Here's how the part is built. I have some questions about the finished solid (model axes, mm). A direction names the side the tool comes from. Round coordinates to 2 decimals unless told otherwise and drop trailing zeros. Order: outer loops, then holes, each group sorted by start corner. A loop starts at its lowest first (then second) coordinate and runs counter-clockwise, first axis right, second up. Notation, with made-up numbers: (-26.5, -7.75) - (18.5, -7.75) arc R10 cw to (18.5, 2.25) - close; hole circle Ø5 at (68.25, -18). An arc over 180 degrees is marked (long way). Answer as a JSON object with one key per item and string values.
```python
from build123d import *

# Parameters (mm, degrees)
SKETCH_W           = 42.3
SKETCH_H           = 42.3
PAD_DEPTH          = 38
SKETCH001_R        = 11.4
PAD001_DEPTH       = 40
SKETCH002_R        = 2.5
PAD002_DEPTH       = 61.5
CHAMFER_SIZE       = 5
SKETCH003_W        = 10
SKETCH003_H        = 3
POCKET_DEPTH       = 18
SKETCH004_W        = 16.2
SKETCH004_H        = 27.15
PAD003_DEPTH       = 9.4
SKETCH005_R        = 2.25
POCKET001_DEPTH    = 4.5
POLARPATTERN_COUNT = 4


with BuildPart() as part:
    # Sketch → Pad (new body)
    with BuildSketch(Plane.XY):
        Rectangle(SKETCH_W, SKETCH_H)
    extrude(amount=PAD_DEPTH)

    # Sketch001 → Pad001 (join)
    with BuildSketch(Plane.XY):
        Circle(SKETCH001_R)
    extrude(amount=PAD001_DEPTH)

    # Sketch002 → Pad002 (join)
    with BuildSketch(Plane.XY):
        Circle(SKETCH002_R)
    extrude(amount=PAD002_DEPTH)

    # Chamfer
    chamfer_edges = [part.edges().sort_by_distance(p)[0] for p in [
        (-21.15, 21.15, 19),
        (-21.15, -21.15, 19),
        (21.15, 21.15, 19),
        (21.15, -21.15, 19),
    ]]
    chamfer(chamfer_edges, length=CHAMFER_SIZE)

    # Sketch003 (on Face16 of Chamfer) → Pocket (cut)
    with BuildSketch(Plane.XY.offset(61.5)):
        with Locations((0, 3.5)):
            Rectangle(SKETCH003_W, SKETCH003_H)
    extrude(amount=-POCKET_DEPTH, mode=Mode.SUBTRACT)

    # Sketch004 → Pad003 (join)
    with BuildSketch(Plane.XY):
        with Locations((0, 13.575)):
            Rectangle(SKETCH004_W, SKETCH004_H)
    extrude(amount=PAD003_DEPTH)

    # Sketch005 (on Face5 of Pad003) → Pocket001 (cut)
    with BuildSketch(Plane.XY.offset(38)):
        with Locations((-15.5, 16.484926)):
            Circle(SKETCH005_R)
    pocket001 = extrude(amount=-POCKET001_DEPTH, mode=Mode.SUBTRACT)

    # PolarPattern: Pocket001 ×4 about axis
    polarpattern_axis = Axis((0, 0, 38), (0, 0, 1))
    for i in range(1, POLARPATTERN_COUNT):
        add(pocket001.rotate(polarpattern_axis, i * 360 / POLARPATTERN_COUNT), mode=Mode.SUBTRACT)


solid = part.part
```
1. Imagine slicing it at A-A (z = 6). List the corners of the cut face in (x, y) for me, plus the area to 3 significant figures.
Responses:
{"outline": "(-21.15, -16.15) - (-16.15, -21.15) - (16.15, -21.15) - (21.15, -16.15) - (21.15, 16.15) - (16.15, 21.15) - (8.1, 21.15) - (8.1, 27.15) - (-8.1, 27.15) - (-8.1, 21.15) - (-16.15, 21.15) - (-21.15, 16.15) - close", "area": "1,840 mm2"}
2. Imagine slicing it at B-B (y = -10). List the corners of the cut face in (x, z) for me, plus the area to 3 significant figures.
Responses:
{"outline": "(-21.15, 0) - (21.15, 0) - (21.15, 38) - (5.47, 38) - (5.47, 40) - (-5.47, 40) - (-5.47, 38) - (-21.15, 38) - close", "area": "1,630 mm2"}
3. For faces 1 (the face through (0, 2, 53)), 2 (the face through (0, 3, 0)), 3 (the face through (18.38, 14.29, 35.78)), 4 (the face through (8.1, 24, 5)), 5 (the face through (-8.1, 24, 5)), which set-ups out of +Z, -Z, +X, -X, +Y, -Y let a thin tool reach every point of the face, with its end or its side?
Responses:
{"face 1": "+Z, +X, -X, +Y", "face 2": "-Z, +X, -X, +Y, -Y", "face 3": "+Z", "face 4": "+Z, -Z, +X, +Y", "face 5": "+Z, -Z, -X, +Y"}
4. Thinking about a two-plate mould opening in X: for faces 6 (the face through (-17, -16, 33.5)), 7 (the face through (14.29, -18.38, 35.78)), 8 (the face through (9, -9, 38)), 9 (the face through (18.7, 18.6, 18.7)), which applies, pulls with the +X half, pulls with the -X half, needs draft (parallel to the pull), parting line crosses it, or undercut?
Responses:
{"face 6": "undercut", "face 7": "undercut", "face 8": "needs draft", "face 9": "pulls with the +X half"}
5. For P1, Ø1.8, axis at x = -1.5, y = 23, coming from the +Z side; P2, Ø3.5, axis at x = 0.5, z = 53, coming from the +Y side; P3, Ø1.5, axis at x = -3.5, y = 9, coming from the +Z side; P4, Ø5, axis at y = 5.5, z = 54.5, coming from the +X side, each with a flat end and sliding along its axis, tell me the tip position at first contact or that it passes through.
Responses:
{"P1": "z = 9.4", "P2": "y = 2", "P3": "z = 40", "P4": "through"}
6. Imagine slicing it at C-C (x = 0). List the corners of the cut face in (y, z) for me.
Responses:
{"outline": "(-21.15, 0) - (27.15, 0) - (27.15, 9.4) - (21.15, 9.4) - (21.15, 38) - (11.4, 38) - (11.4, 40) - (2.5, 40) - (2.5, 43.5) - (2, 43.5) - (2, 61.5) - (-2.5, 61.5) - (-2.5, 40) - (-11.4, 40) - (-11.4, 38) - (-21.15, 38) - close"}
7. If I drill on L1, parallel to Y at x = -17.5, z = 34; L2, parallel to X at y = -15, z = 36; L3, parallel to Z at x = 16, y = -4, over which ranges is the centre line in solid material (lowest first)? Write a range as [from, to].
Responses:
{"L1": "[-19.8, -17.51], [-13.49, 15.45], [17.52, 19.8]", "L2": "[-21.15, -18.68], [-14.29, 13.81], [17.19, 21.15]", "L3": "[0, 38]"}
8. Imagine slicing it at D-D (y = -4). List the corners of the cut face in (x, z) for me.
Responses:
{"outline": "(-21.15, 0) - (21.15, 0) - (21.15, 38) - (10.68, 38) - (10.68, 40) - (-10.68, 40) - (-10.68, 38) - (-21.15, 38) - close"}
